from build123d import *

# Parameters (mm, degrees)
AUFSATZ_LINEAR_AUSTRAGEN1_DEPTH = 15.2
SKIZZE2_R                       = 2.5
AUFSATZ_LINEAR_AUSTRAGEN2_DEPTH = 1.3
SKIZZE3_R                       = 0.5
AUFSATZ_LINEAR_AUSTRAGEN3_DEPTH = 2
VERRUNDUNG1_R                   = 0.2
SKIZZE4_W                       = 0.3
SKIZZE4_H                       = 4.8
SCHNITT_LINEAR_AUSTRAGEN1_DEPTH = 0.1
SKIZZE5_W                       = 0.3
SKIZZE5_H                       = 1.5
AUFSATZ_LINEAR_AUSTRAGEN4_DEPTH = 1.7
SCHNITT_LINEAR_AUSTRAGEN2_REACH = 22.19
SKIZZE6_R                       = 0.3
VERRUNDUNG2_R                   = 0.2


with BuildPart() as part:
    # Skizze1 → Aufsatz-Linear austragen1 (new body)
    with BuildSketch(Plane.XY):
        with BuildLine():
            Line((-3.31662479, 5), (3.31662479, 5))
            ThreePointArc((3.31662479, 5), (6, 0), (3.31662479, -5))
            Line((3.31662479, -5), (-3.31662479, -5))
            ThreePointArc((-3.31662479, -5), (-6, 0), (-3.31662479, 5))
        make_face()
    extrude(amount=AUFSATZ_LINEAR_AUSTRAGEN1_DEPTH)

    # Skizze2 → Aufsatz-Linear austragen2 (add)
    with BuildSketch(Plane.XY.offset(15.2)):
        Circle(SKIZZE2_R)
    extrude(amount=AUFSATZ_LINEAR_AUSTRAGEN2_DEPTH)

    # Skizze3 → Aufsatz-Linear austragen3 (add)
    with BuildSketch(Plane(origin=(0, 0, 0), x_dir=(-1, 0, 0), z_dir=(0, 0, -1))):
        with Locations(Location((0, 0, 0), (0, 0, 180))):
            Circle(SKIZZE3_R)
    extrude(amount=AUFSATZ_LINEAR_AUSTRAGEN3_DEPTH)

    # Verrundung1
    verrundung1_edges = [part.edges().sort_by_distance(p)[0] for p in [
        (6, 0, 15.2),
        (0, 5, 15.2),
        (-2.5, 0, 16.5),
        (-6, 0, 15.2),
        (0, 5, 0),
        (6, 0, 0),
        (0, -5, 0),
        (-6, 0, 0),
        (0, -5, 15.2),
    ]]
    fillet(verrundung1_edges, radius=VERRUNDUNG1_R)

    # Skizze4 → Schnitt-Linear austragen1 (cut)
    with BuildSketch(Plane(origin=(0, 5, 0), x_dir=(1, 0, 0), z_dir=(0, 1, 0))):
        with Locations((-2.15, -6.8)):
            Rectangle(SKIZZE4_W, SKIZZE4_H)
        with Locations((2.15, -6.8)):
            Rectangle(SKIZZE4_W, SKIZZE4_H)
    schnitt_linear_austragen1 = extrude(amount=-SCHNITT_LINEAR_AUSTRAGEN1_DEPTH, mode=Mode.SUBTRACT)

    # Spiegeln1: Schnitt-Linear austragen1 across plane
    add(schnitt_linear_austragen1.mirror(Plane.ZX), mode=Mode.SUBTRACT)

    # Skizze5 → Aufsatz-Linear austragen4 (add)
    with BuildSketch(Plane.XY.offset(15.2)):
        with Locations((-3.7, 0)):
            Rectangle(SKIZZE5_W, SKIZZE5_H)
        with Locations((3.7, 0)):
            Rectangle(SKIZZE5_W, SKIZZE5_H)
    extrude(amount=AUFSATZ_LINEAR_AUSTRAGEN4_DEPTH)

    # Skizze6 → Schnitt-Linear austragen2 (cut, up to next)
    with BuildSketch(Plane.ZY.offset(3.85), mode=Mode.PRIVATE) as schnitt_linear_austragen2_sk1:
        with Locations((16.2, 0)):
            Circle(SKIZZE6_R)
    schnitt_linear_austragen2_tool1 = extrude(schnitt_linear_austragen2_sk1.sketch, amount=-SCHNITT_LINEAR_AUSTRAGEN2_REACH, mode=Mode.PRIVATE) & part.part
    schnitt_linear_austragen2 = schnitt_linear_austragen2_tool1.solids().sort_by_distance((-3.85, 0, 16.2))[0]
    add(schnitt_linear_austragen2, mode=Mode.SUBTRACT)

    # Spiegeln6: Schnitt-Linear austragen2 across plane
    add(schnitt_linear_austragen2.mirror(Plane(origin=(0, 0, 0), x_dir=(0, 0, 1), z_dir=(1, 0, 0))), mode=Mode.SUBTRACT)

    # Verrundung2
    verrundung2_edges = [part.edges().sort_by_distance(p)[0] for p in [
        (-3.7, -0.75, 16.9),
        (-3.7, 0.75, 16.9),
        (3.7, -0.75, 16.9),
        (3.7, 0.75, 16.9),
    ]]
    fillet(verrundung2_edges, radius=VERRUNDUNG2_R)


solid = part.part
Here's how the part is built. I have some questions about the finished solid (model axes, mm). A direction names the side the tool comes from. Coordinates: 2 decimals unless noted, no trailing zeros. Loops run counter-clockwise (first coordinate to the right, second up) from the corner with the lowest first, then second, coordinate; pieces in that order, holes last.
1. If we mould it in two halves opening along X, with no side actions, what happens to faces 4 (the flat face through (0, 0, 16.5)), 5 (the flat face through (0, -5, 7)), 6 (the flat face through (-3.85, 0, 15.7))? For each: pulls with the +X half, pulls with the -X half, needs draft (parallel to the pull), parting line crosses it, or undercut.
2. Imagine slicing it at C-C, the plane z = 3. Please give me the cut outline in (x, y).
3. For P1, Ø0.8, axis at y = 0, z = 16, coming from the +X side; P2, Ø3, axis at y = -2, z = 7.5, coming from the +X side; P3, Ø1, axis at y = -3, z = 11, coming from the +X side; P4, Ø6, axis at y = -2, z = 1, coming from the -X side, each with a flat end and sliding along its axis, tell me the tip position at first contact or that it passes through.
4. Imagine slicing it at B-B, the plane x = 0. Please give me the cut outline in (y, z), and give its area (3 significant figures).
5. For faces 1 (the cylindrical face through (-0.108, 0.488, -0.986)), 2 (the flat face through (-3.55, 0, 15.7)), 3 (the flat face through (3, 0, 15.2)), which set-ups out of +Z, -Z, +X, -X, +Y, -Y let a thin tool reach every point of the face, with its end or its side?
6. I need wall thicknesses on L1, parallel to Y at x = -3.7, z = 16.2; L2, parallel to Z at x = -1, y = 4; L3, parallel to Z at x = 1.75, y = 0. Which ranges of each line are inside material? Lowest first, please.
7. Imagine slicing it at A-A, the plane y = 0. Count the separate pieces of the cut face and the enclosed holes in it, and give its area (3 significant figures).
Taken from the geometry:
1. face 4: undercut
1. face 5: needs draft
1. face 6: pulls with the -X half
2. outline: (-3.32, -5) - (3.32, -5) arc R6 ccw to (3.32, 5) - (-3.32, 5) arc R6 ccw to start
3. P1: stops at x = 3.85
3. P2: stops at x = 5.98
3. P3: stops at x = 5.45
3. P4: stops at x = -6
4. outline: (-5, 0.2) arc R0.2 ccw to (-4.8, 0) - (-0.5, 0) - (-0.5, -2) - (0.5, -2) - (0.5, 0) - (4.8, 0) arc R0.2 ccw to (5, 0.2) - (5, 15) arc R0.2 ccw to (4.8, 15.2) - (2.5, 15.2) - (2.5, 16.3) arc R0.2 ccw to (2.3, 16.5) - (-2.3, 16.5) arc R0.2 ccw to (-2.5, 16.3) - (-2.5, 15.2) - (-4.8, 15.2) arc R0.2 ccw to (-5, 15) - close
4. area: 160 mm2
5. face 1: -Z
5. face 2: +Z, +Y, -Y
5. face 3: +Z
6. L1: y = -0.75 to -0.3, 0.3 to 0.75
6. L2: z = 0 to 15.2
6. L3: z = 0 to 16.5
7. separate pieces: 3
7. enclosed holes: 0
7. area: 192 mm2
